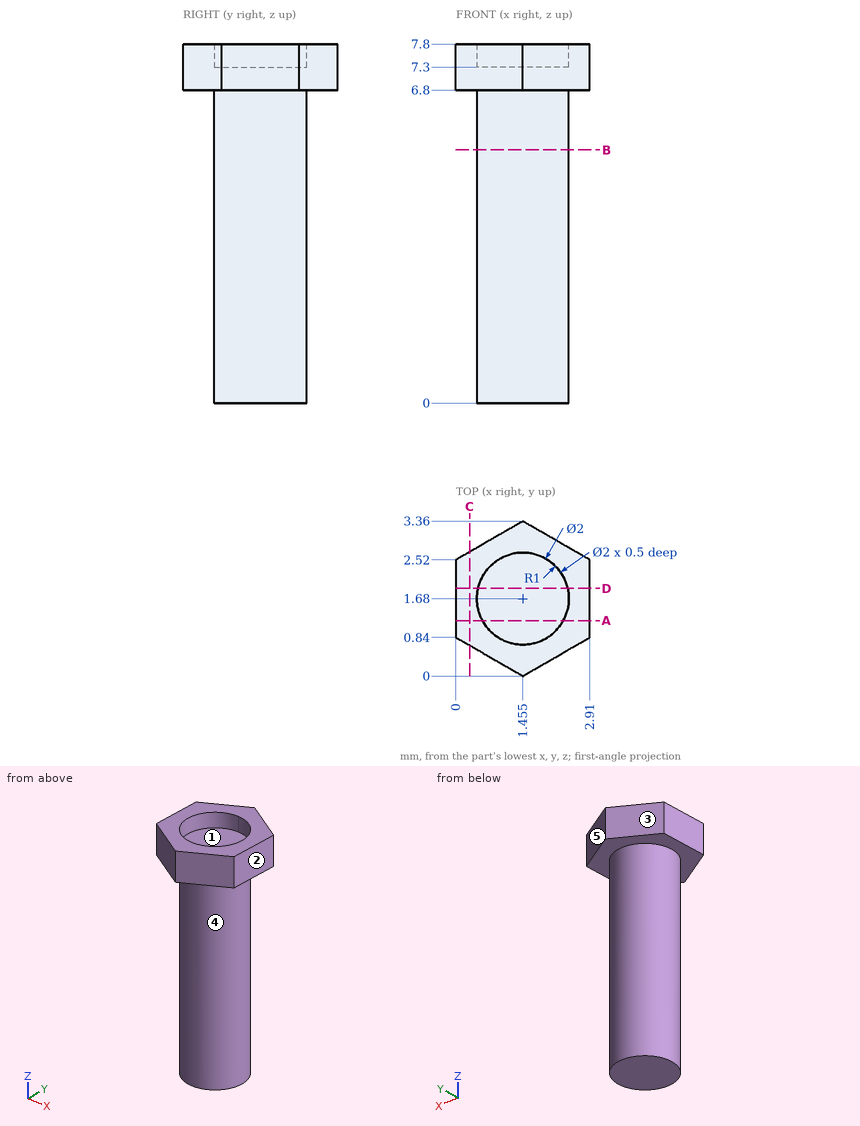
Design review of the part shown in the three views and the two pictorial views. Dimensions are in mm from the part's minimum x, y and z. A direction names the side the tool comes from. Round coordinates to 2 decimals unless told otherwise and drop trailing zeros. Write each loop counter-clockwise with the first axis right and the second up, starting at its lowest first coordinate (ties: lowest second). Pieces come first, ordered by that corner, then holes.
Item 1: We need section C-C on x = 0.3. Write out the cut boundary in (y, z).
Item 2: We need section A-A on y = 1.2. Write out the cut boundary in (x, z), and give its area (3 significant figures).
Item 3: Clearance check with flat-ended pins moving along their axes: pin 1 Ø1.5 at (x, y) = (1, 2) entering from -Z; pin 2 Ø1 at (y, z) = (2.5, 2) entering from +X; pin 3 Ø1.5 at (y, z) = (1.5, 5.5) entering from -X (3 decimals). State where each tip first meets the part, or that it passes through.
Item 4: For probe 1 along X at (y, z) = (1.68, 7.45) (3 decimals); probe 2 along Z at (x, y) = (2.1, 2.9); probe 3 along Y at (x, z) = (1.5, 4.75), list the stretches that pass through material, from the lowest coordinate up.
Item 5: For the marked faces 4 and 5, list the 3-axis set-ups (+Z, -Z, +X, -X, +Y, -Y) from which the entire face can be reached by the end or side of a thin tool; tool diameter is ignored.
Item 6: We need section D-D on y = 1.9. Write out the cut boundary in (x, z).
Item 7: The part is to be moulded in two halves that separate along X. For the marked faces 1, 2 and 3, say which applies: +X half, -X half, draft (parallel to the pull), parting line (faces both ways), or undercut.
Item 8: We need section B-B on z = 5.5. Write out the cut boundary in (x, y) (3 decimals).
Returned:
1. outline: (0.67, 6.8) - (2.69, 6.8) - (2.69, 7.8) - (0.67, 7.8) - close
2. outline: (0, 6.8) - (0.58, 6.8) - (0.58, 0) - (2.33, 0) - (2.33, 6.8) - (2.91, 6.8) - (2.91, 7.8) - (2.33, 7.8) - (2.33, 7.3) - (0.58, 7.3) - (0.58, 7.8) - (0, 7.8) - close
2. area: 14.0 mm2
3. pin 1: stops at z = 0
3. pin 2: stops at x = 2.4
3. pin 3: stops at x = 0.455
4. probe 1: x = 0 to 0.455, 2.455 to 2.91
4. probe 2: z = 6.8 to 7.8
4. probe 3: y = 0.68 to 2.68
5. face 4: -Z
5. face 5: +Z, -Z, +X, +Y
6. outline: (0, 6.8) - (0.48, 6.8) - (0.48, 0) - (2.43, 0) - (2.43, 6.8) - (2.91, 6.8) - (2.91, 7.8) - (2.43, 7.8) - (2.43, 7.3) - (0.48, 7.3) - (0.48, 7.8) - (0, 7.8) - close
7. face 1: undercut
7. face 2: +X half
7. face 3: -X half
8. outline: circle Ø2 at (1.455, 1.68)
